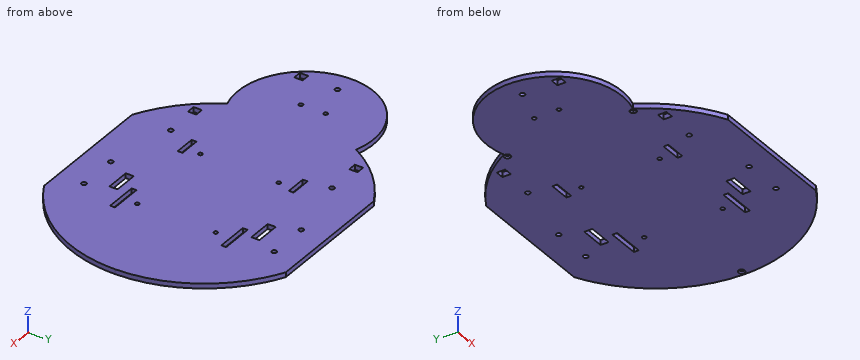
Autodesk Inventor part; units mm, degrees
ref_plane "YZ Plane" through (0, 0, 0) normal (1, 0, 0) x (0, 1, 0)
ref_plane "XZ Plane" through (0, 0, 0) normal (0, 1, 0) x (-1, 0, 0)
ref_plane "XY Plane" through (0, 0, 0) normal (0, 0, 1) x (1, 0, 0)
sketch "Base" plane through (0, 0, 0) normal (0, 0, 1) x (1, 0, 0)
  circle A0 centre (-28.7523, 24.2466) radius 1.25
  circle A1 centre (-29.1949, -24.7514) radius 1.25
  arc A2 (-77.2059, 40) -> (-77.2059, -40) centre (-90.3849, 0) ccw
  line L0 (41.0629, -75.0587) -> (-41.0629, -75.0587)
  ellipse E0 centre (0, 0) end of major axis (-87.5, 0) minor radius 85 (-77.2059, -40) -> (-41.0629, -75.0587) ccw
  line L1 (0, 0) -> (87.5, 0)
  line L2 (41.0629, 75.0587) -> (-41.0629, 75.0587)
  ellipse E1 centre (0, 0) end of major axis (-87.5, 0) minor radius 85 (41.0629, -75.0587) -> (41.0629, 75.0587) ccw
  ellipse E2 centre (0, 0) end of major axis (-87.5, 0) minor radius 85 (-41.0629, 75.0587) -> (-77.2059, 40) ccw
  circle A3 centre (29.2453, 23.7226) radius 1.25
  circle A4 centre (28.8027, -25.2754) radius 1.25
  dimension "d84" = 87.5
  dimension "d85" = 75.0587
  dimension "d88" = 42.1151
sketch "Holes and Mounts" plane through (0, 0, 0) normal (0, 0, 1) x (1, 0, 0)
  line L0 (-9.7798, -74.0877) -> (40.2202, -74.0877)
  circle A0 centre (2.62, -59.0877) radius 1.5
  circle A1 centre (27.82, -59.0877) radius 1.5
  circle A2 centre (-39.757, 45.9313) radius 1.5
  line L1 (-59.657, 43.3313) -> (-64.857, 43.3313)
  line L2 (-64.857, 43.3313) -> (-64.857, 48.5313)
  line L3 (-64.857, 48.5313) -> (-59.657, 48.5313)
  line L4 (-59.657, 48.5313) -> (-59.657, 43.3313)
  line L5 (-59.657, 43.3313) -> (-64.857, 48.5313) construction
  line L6 (-64.857, 43.3313) -> (-59.657, 48.5313) construction
  line L7 (-9.7798, -74.0877) -> (-9.7798, -44.0877)
  line L8 (-9.7798, -44.0877) -> (40.2202, -44.0877)
  line L9 (40.2202, -44.0877) -> (40.2202, -74.0877)
  line L10 (59.2442, -0.0127) -> (-26.2941, -0.0127)
  circle A3 centre (2.62, 59.0622) radius 1.5
  circle A4 centre (27.82, 59.0622) radius 1.5
  line L11 (-9.7798, 74.0622) -> (40.2202, 74.0622)
  line L12 (-9.7798, 44.0622) -> (40.2202, 44.0622)
  line L13 (40.2202, 74.0622) -> (40.2202, 44.0622)
  line L14 (-9.7798, 74.0622) -> (-9.7798, 44.0622)
  circle A5 centre (-39.757, -45.9568) radius 1.5
  line L15 (-59.657, -48.5568) -> (-59.657, -43.3568)
  line L16 (-64.857, -48.5568) -> (-59.657, -48.5568)
  line L17 (-59.657, -43.3568) -> (-64.857, -43.3568)
  line L18 (-64.857, -43.3568) -> (-64.857, -48.5568)
  line L19 (-59.657, -43.3568) -> (-64.857, -48.5568) construction
  line L20 (-64.857, -43.3568) -> (-59.657, -48.5568) construction
  dimension "d53" = 3
  dimension "d54" = 5.2
  dimension "d55" = 5.2
  dimension "d62" = 30
extrude "ComponentARBHoles" add sketch "Base" along normal blind 3
sketch "Holes Only" plane through (0, 0, 3) normal (0, 0, 1) x (1, 0, 0)
  line L0 (-117.446, -25.0998) -> (-117.446, -19.8998)
  line L1 (-117.446, -19.8998) -> (-122.646, -19.8998)
  line L2 (-122.646, -19.8998) -> (-122.646, -25.0998)
  circle A0 centre (-120.046, 0.0002) radius 1.5
  line L3 (-122.646, -25.0998) -> (-117.446, -25.0998)
  circle A1 centre (27.82, -59.0877) radius 1.5
  line L4 (27.82, -59.0877) -> (2.62, -59.0877)
  circle A2 centre (27.82, -59.0877) radius 1.5
  circle A3 centre (2.62, -59.0877) radius 1.5
  circle A4 centre (2.62, -59.0877) radius 1.5
  circle A5 centre (2.62, 59.0622) radius 1.5
  line L5 (2.62, 59.0622) -> (27.82, 59.0622)
  circle A6 centre (2.62, 59.0622) radius 1.5
  circle A7 centre (27.82, 59.0622) radius 1.5
  point P0 (0, 0)
extrude "WheelFrontSensorHoles" cut sketch "Holes Only" against normal blind 10
sketch "SensorHolesSidesSketch" plane through (0, 0, 0) normal (0, 0, -1) x (-1, 0, 0)
  circle A0 centre (39.757, -50.0587) radius 1.5
  line L0 (64.857, -52.6587) -> (59.657, -52.6587)
  line L1 (64.857, -47.4587) -> (64.857, -52.6587)
  line L2 (59.657, -47.4587) -> (64.857, -47.4587)
  line L3 (59.657, -52.6587) -> (59.657, -47.4587)
  circle A1 centre (39.757, -50.0587) radius 1.5
  line L4 (64.857, -52.6587) -> (59.657, -52.6587)
  line L5 (59.657, -52.6587) -> (59.657, -47.4587)
  line L6 (59.657, -47.4587) -> (64.857, -47.4587)
  line L7 (64.857, -47.4587) -> (64.857, -52.6587)
  line L8 (39.757, -45.9568) -> (39.757, -75.0587)
  line L9 (41.0629, -75.0587) -> (-41.0629, -75.0587)
  line L10 (39.757, -75.0587) -> (39.757, -50.0587)
  point P0 (0, 0)
  point P1 (39.757, 45.9313)
  point P2 (59.657, 48.5313)
sketch "Sketch9" plane through (0, 0, 3) normal (0, 0, 1) x (1, 0, 0)
  point P0 (0, 0)
sketch "HolderSlotsSketch" plane through (0, 0, 0) normal (0, 0, -1) x (-1, 0, 0)
  line L0 (-41.0629, 75.0587) -> (41.0629, 75.0587)
  line L1 (22.9567, 75.0587) -> (-16.4493, 75.0587)
  line L2 (0, 0) -> (-128.8133, 0)
  line L3 (0, 0) -> (-38, 0)
  line L4 (-38, 33) -> (-38, 36)
  line L5 (-38, 36) -> (-18, 36)
  line L6 (25, 36) -> (38, 36)
  line L7 (38, 36) -> (38, 33)
  line L8 (38, 0) -> (0, 0)
  line L9 (-38, 36) -> (-18, 36)
  line L10 (-18, 36) -> (-18, 33)
  line L11 (-18, 33) -> (-38, 33)
  line L12 (-38, 33) -> (-38, 36)
  line L13 (38, 36) -> (25, 36)
  line L14 (25, 36) -> (25, 33)
  line L15 (25, 33) -> (38, 33)
  line L16 (38, 33) -> (38, 36)
  line L17 (-38, -33) -> (-38, -36)
  line L18 (-38, -36) -> (-18, -36)
  line L19 (25, -36) -> (38, -36)
  line L20 (38, -36) -> (38, -33)
  line L21 (-38, -36) -> (-18, -36)
  line L22 (-18, -36) -> (-18, -33)
  line L23 (-18, -33) -> (-38, -33)
  line L24 (-38, -33) -> (-38, -36)
  line L25 (38, -36) -> (25, -36)
  line L26 (25, -36) -> (25, -33)
  line L27 (25, -33) -> (38, -33)
  line L28 (38, -33) -> (38, -36)
extrude "HolderSlots" cut sketch "HolderSlotsSketch" against normal blind 10
sketch "Sketch11" plane through (0, 0, 0) normal (0, 0, -1) x (-1, 0, 0)
  ellipse E0 centre (0, 0) end of major axis (87.5, 0) minor radius 85 (-41.0629, 75.0587) -> (-41.0629, -75.0587) ccw
  circle A0 centre (0, 0) radius 81.5
  line L0 (-81.5, 0) -> (-87.5, 0)
  line L1 (-81.5, 0) -> (-84.5, 0)
  circle A1 centre (-84.5, 0) radius 3
  circle A2 centre (-84.5, 0) radius 2
  dimension "d100" = 163
  dimension "d101" = 4
extrude "MagnetHoleBottom" cut sketch "Sketch11" against normal blind 1.5 contours A2 L0 | L0 A2
sketch "Sketch13" plane through (0, 0, 0) normal (0, 0, -1) x (-1, 0, 0)
  circle A0 centre (74.8228, 39.4351) radius 2
  circle A1 centre (74.98, -38.7948) radius 2
  circle A2 centre (74.98, -38.7948) radius 2
  circle A3 centre (74.8228, 39.4351) radius 2
  point P0 (0, 0)
extrude "MagnetHoleSides" cut sketch "Sketch13" against normal blind 1.5
sketch "Sketch14" plane through (0, 0, 0) normal (0, 0, -1) x (-1, 0, 0)
  circle A0 centre (-27.82, 59.0622) radius 1.5 construction
  circle A1 centre (-2.62, 59.0622) radius 1.5 construction
  line L0 (-7.62, 45.0622) -> (-7.62, 41.5622)
  line L1 (-7.62, 41.5622) -> (-22.82, 41.5622)
  line L2 (-22.82, 41.5622) -> (-22.82, 44.0622)
  line L3 (-7.62, 45.0622) -> (-7.62, 46.5622)
  line L4 (-7.62, 46.5622) -> (-22.82, 46.5622)
  line L5 (-22.82, 46.5622) -> (-22.82, 44.0622)
  point P0 (0, 0)
  dimension "d120" = 2.5
  dimension "d121" = 2.5
extrude "Extrusion10" cut sketch "Sketch14" against normal blind 10
mirror "Mirror2" about plane through (0, 0, 0) normal (0, 1, 0) of "Extrusion10"
sketch "Sketch15" plane through (0, 0, 0) normal (0, 0, -1) x (-1, 0, 0)
  circle A0 centre (97.5, 7.7) radius 1.27
  circle A1 centre (97.5, -7.7) radius 1.27
  line L0 (-41.4439, -82.7587) -> (-41.4439, -75.0587)
  arc A2 (77.2059, -40) -> (77.2059, 40) centre (90.3849, 0) ccw
  point P0 (0, 0)
  dimension "d122" = 2.54
  dimension "d123" = 2.54
extrude "Ball Caster Holes" cut sketch "Sketch15" against normal blind 10
extrude "Extrusion12" cut sketch "SensorHolesSidesSketch" against normal blind 10
mirror "Mirror3" about plane through (0, 0, 0) normal (0, 1, 0) of "Extrusion12"
properties part number "Base component"
The model under review builds one solid part; all positions refer to its coordinate system, in mm. Round coordinates to 2 decimals unless told otherwise and drop trailing zeros. Order: outer loops, then holes, each group sorted by start corner. A loop starts at its lowest first (then second) coordinate and runs counter-clockwise, first axis right, second up. Notation, with made-up numbers: (-19.5, -30) -> (30.5, -30) arc R8 ccw to (30.5, -24) -> close; hole circle Ø1 at (89.25, 78.25). An arc over 180 degrees is marked (long way). Write item = value, one per line. Start each with the question number.
Item 1: For line 1 along Y through (x, z) = (3, 2.4); line 2 along Y through (x, z) = (22, 2); line 3 along Y through (x, z) = (-74.98, 0.7), list the stretches that pass through material, from the lowest coordinate up.
Item 2: Consider section B-B on z = 2. Count the separate pieces of the cut face and the enclosed holes in it, plus the area to 3 significant figures.
Item 3: Consider section A-A on x = 33.5. Write out the cut boundary in (y, z).
Item 4: Clearance check with flat-ended pins moving along their axes: pin 1 Ø3 at (x, y) = (84.5, 0) entering from -Z; pin 2 Ø1 at (y, z) = (9.5, 2.5) entering from -X; pin 3 Ø0.9 at (y, z) = (-34.5, 1.5) entering from -X. State where each tip first meets the part, or that it passes through.
Conclusion:
q1.line_1 = -75.06 to -60.54, -57.64 to 57.61, 60.51 to 75.06
q1.line_2 = -75.06 to -46.56, -41.56 to -36, -33 to 33, 36 to 41.56, 46.56 to 75.06
q1.line_3 = -43.81 to -40.79, -36.79 to 37.44, 41.43 to 43.81
q2.separate_pieces = 1
q2.enclosed_holes = 22
q2.area = 25,100 mm2
q3.outline = (-75.06, 0) -> (-36, 0) -> (-36, 3) -> (-75.06, 3) -> close; (-33, 0) -> (33, 0) -> (33, 3) -> (-33, 3) -> close; (36, 0) -> (75.06, 0) -> (75.06, 3) -> (36, 3) -> close
q4.pin_1 = 1.5
q4.pin_2 = -131.53
q4.pin_3 = -115.17
